Work out the finished part from the listing and answer in its coordinate system (mm). Give positions to 0.01 mm unless a question says otherwise; leave off trailing zeros. Write item = value, one per line.
from build123d import *

# Parameters (mm, degrees)
SKETCH1_W           = 146
SKETCH1_H           = 48
SKETCH1_R           = 1.5
BOSS_EXTRUDE1_DEPTH = 3
FILLET1_R           = 2


with BuildPart() as part:
    # Sketch1 → Boss-Extrude1 (new body)
    with BuildSketch(Plane.XY):
        with Locations((73, 24)):
            Rectangle(SKETCH1_W, SKETCH1_H)
        with Locations((3, 45)):
            Circle(SKETCH1_R, mode=Mode.SUBTRACT)
        with Locations((3, 3)):
            Circle(SKETCH1_R, mode=Mode.SUBTRACT)
        with Locations((143, 45)):
            Circle(SKETCH1_R, mode=Mode.SUBTRACT)
        with Locations((143, 3)):
            Circle(SKETCH1_R, mode=Mode.SUBTRACT)
    extrude(amount=BOSS_EXTRUDE1_DEPTH)

    # Fillet1
    fillet1_edges = [part.edges().sort_by_distance(p)[0] for p in [
        (0, 0, 1.5),
        (0, 48, 1.5),
        (146, 48, 1.5),
        (146, 0, 1.5),
    ]]
    fillet(fillet1_edges, radius=FILLET1_R)


solid = part.part
1. A straight line is drawn through the part: line 1 (Y direction, x = 3, z = 0.85). Find the intervals that lie inside material, in ascending order.
Solution:
line_1 = 0 to 1.5, 4.5 to 43.5, 46.5 to 48
2. Given pin 1 (12 mm diameter, centred on x = 88, y = 27, fed in from -Z), flat-ended and moving along its own axis, determine where the tip first touches the part or whether it passes through.
Solution:
pin_1 = 0
3. For a pull along Y with two mould halves and no side action, classify faces 1 (the cylindrical face through (3.69, 1.67, 1.48)), 2 (the flat face through (72, 0, 1)), 3 (the flat face through (0, 24, 1)), 4 (the cylindrical face through (141.5, 3.07, 1.48)) as pulls with the +Y half, pulls with the -Y half, needs draft (parallel to the pull), parting line crosses it, or undercut.
Solution:
face_1 = undercut
face_2 = pulls with the -Y half
face_3 = needs draft
face_4 = undercut
